Answer from the drawing. Dimensions are ordinates in mm from the lowest x, y and z of the part. Give positions to 0.01 mm unless a question says otherwise; leave off trailing zeros. Loops run counter-clockwise (first coordinate to the right, second up) from the corner with the lowest first, then second, coordinate; pieces in that order, holes last. Notation, with made-up numbers: M 74,8 L 90,8 A32 cw 90,41 Z; hole C 7,66.25 d7. An arc over 180 degrees is marked long. Use a Markdown table: item, result.
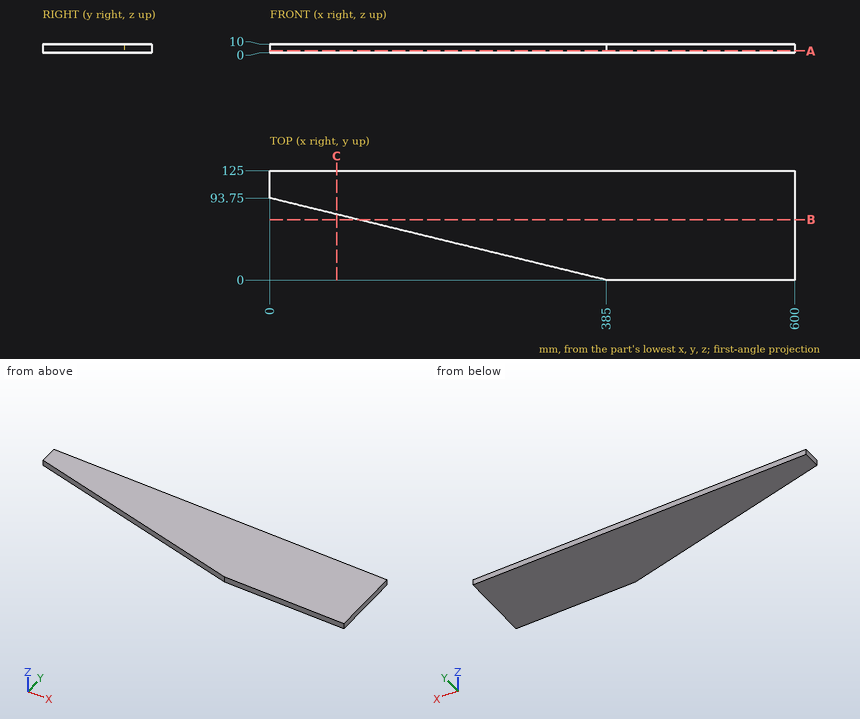
(1) Consider probe 1 along Y at (x, z) = (213.5, 1.5); probe 2 along Y at (x, z) = (247, 4). Determine where each line is inside the solid, lowest interval first. Write a range as [from, to].
Entries:
| item | result |
|---|---|
| probe 1 | y = [41.76, 125] |
| probe 2 | y = [33.6, 125] |
(2) A cutting plane is placed at A-A (z = 2.25). Write down the section's boundary in (x, y), and give its area (3 significant figures).
Entries:
| item | result |
|---|---|
| outline | M 0,93.75 L 385,0 L 600,0 L 600,125 L 0,125 Z |
| area | 57,000 mm² |
(3) A cutting plane is placed at C-C (x = 76.5). Write down the section's boundary in (y, z).
Entries:
| item | result |
|---|---|
| outline | M 75.12,0 L 125,0 L 125,10 L 75.12,10 Z |
(4) Given P1, Ø5, axis at x = 148, z = 7, coming from the -Y side; P2, Ø1, axis at y = 108.5, z = 6, coming from the -X side; P3, Ø5, axis at x = 171.5, z = 6.5, coming from the -Y side, each flat-ended and moving along its own axis, determine where each tip first touches the part or whether it passes through.
Entries:
| item | result |
|---|---|
| P1 | stops at y = 57.1 |
| P2 | stops at x = 0 |
| P3 | stops at y = 51.38 |
(5) A cutting plane is placed at B-B (y = 69). Write down the section's boundary in (x, z).
Entries:
| item | result |
|---|---|
| outline | M 101.64,0 L 600,0 L 600,10 L 101.64,10 Z |
